Geometry: final body of the model. Coordinates: model frame, mm. Face numbers are marked on the shaded views. A direction names the side the tool comes from. Give positions to 0.01 mm unless a question says otherwise; leave off trailing zeros. Write each loop counter-clockwise with the first axis right and the second up, starting at its lowest first coordinate (ties: lowest second). Pieces come first, ordered by that corner, then holes. Notation, with made-up numbers: M -18,66 L 1,66 A17 cw 1,76 Z; hole C 9.25,-9.5 d7. An arc over 180 degrees is marked long. Use a Markdown table: item, result. Add a question column.
(1) Material intervals for L1, parallel to X at y = -2.5, z = 3; L2, parallel to X at y = 0, z = 2.5; L3, parallel to Z at x = 6.5, y = -3.5, sorted ascending.
(2) Pin query (flat end, axial travel): pin 1 Ø1 at (x, y) = (-14.5, -1.5) entering from -Z; pin 2 Ø8 at (x, z) = (20.5, 21.5) entering from -Y; pin 3 Ø1 at (x, z) = (-3.5, 25.5) entering from +Y; pin 4 Ø10 at (x, z) = (-38, 12) entering from +Y. Return the tip coordinate at first contact, or that it passes through.
(3) Cut plane A-A (y = 0). Output: boundary loops of the cut face in (x, z), plus the area to 3 significant figures.
(4) Cut plane C-C (z = 4). State how many separate pieces and enclosed holes the cut face has, plus the area to 3 significant figures.
(5) Cut plane B-B (x = -1.5). Output: boundary loops of the cut face in (y, z).
(6) Draft query along X for the marked faces 3, 4 and 5. Return one class per face: released by +X, released by -X, zero draft, split by the parting line, or undercut.
(7) Reachability of the marked faces 1 and 2 from +Z, -Z, +X, -X, +Y, -Y: full face, straight path, thin tool, end or side. Return the list, or none.
```python
from build123d import *

# Parameters (mm, degrees)
BOSS_EXTRUDE1_DEPTH             = 6.35
FILLET1_R                       = 6.35
CHAMFER1_SIZE                   = 2
SKETCH3_R                       = 2.54
CUT_EXTRUDE1_DEPTH              = 63.891530963
F_10_CLEARANCE_HOLE1_AT_2_COUNT = 2
F_10_CLEARANCE_HOLE1_AT_2_PITCH = 101.605909567
SKETCH6_R                       = 3.81
CUT_EXTRUDE2_DEPTH              = 63.891531054


with BuildPart() as part:
    # Sketch2 → Boss-Extrude1 (new, symmetric)
    with BuildSketch(Plane(origin=(0, 0, 0), x_dir=(1, 0, 0), z_dir=(0, 1, 0))):
        with BuildLine():
            Line((-27.740386752, -38.1), (27.740386752, -38.1))
            ThreePointArc((27.740386752, -38.1), (48.067233392, -23.381874086), (57.182708636, 0))
            Line((57.182708636, 0), (44.417291364, 0))
            ThreePointArc((44.417291364, 0), (38.295246108, -15.252216058), (25.367291364, -25.4))
            Line((25.367291364, -25.4), (-25.367291364, -25.4))
            ThreePointArc((-25.367291364, -25.4), (-38.295246108, -15.252216058), (-44.417291364, 0))
            Line((-44.417291364, 0), (-57.182708636, 0))
            ThreePointArc((-57.182708636, 0), (-48.067233392, -23.381874086), (-27.740386752, -38.1))
        make_face()
    extrude(amount=BOSS_EXTRUDE1_DEPTH, both=True)

    # Fillet1
    fillet1_edges = [part.edges().sort_by_distance(p)[0] for p in [
        (-25.367291364, 0, 25.4),
        (25.367291364, 0, 25.4),
        (27.740386752, 0, 38.1),
        (-27.740386752, 0, 38.1),
    ]]
    fillet(fillet1_edges, radius=FILLET1_R)

    # Chamfer1
    chamfer1_edges = [part.edges().sort_by_distance(p)[0] for p in [
        (-48.438733528, -6.35, 22.894218644),
        (38.749073181, 6.35, 14.631598188),
        (-38.749073181, -6.35, 14.631598188),
        (-38.749073181, 6.35, 14.631598188),
        (0, -6.35, 25.4),
        (0, 6.35, 25.4),
        (48.438733528, -6.35, 22.894218644),
        (48.438733528, 6.35, 22.894218644),
        (0, -6.35, 38.1),
        (-27.76741166, -6.35, 37.992751984),
        (27.76741166, -6.35, 37.992751984),
        (0, 6.35, 38.1),
        (-27.76741166, 6.35, 37.992751984),
        (27.76741166, 6.35, 37.992751984),
        (-25.4153506, -6.35, 25.238431021),
        (-25.4153506, 6.35, 25.238431021),
        (25.4153506, -6.35, 25.238431021),
        (25.4153506, 6.35, 25.238431021),
        (-48.438733528, 6.35, 22.894218644),
        (38.749073181, -6.35, 14.631598188),
    ]]
    chamfer(chamfer1_edges, length=CHAMFER1_SIZE)

    # Sketch3 → Cut-Extrude1 (cut, through all)
    with BuildSketch(Plane.XY.offset(12.7)):
        with Locations(Location((50.802954783, 0, 0), (0, 0, 180))):
            Circle(SKETCH3_R)
        with Locations(Location((-50.802954783, 0, 0), (0, 0, 180))):
            Circle(SKETCH3_R)
    extrude(amount=CUT_EXTRUDE1_DEPTH, mode=Mode.SUBTRACT)

    # Sketch5 → #10 Clearance Hole1 (revolve, cut)
    with BuildSketch(Plane(origin=(50.802954783, 0, 12.7), x_dir=(0, -1, 0), z_dir=(1, 0, 0))):
        Polygon((0, 0), (0, 12.7), (2.8067, 12.7), (2.8067, 1.0033), (3.81, 0), align=None)
    f_10_clearance_hole1 = revolve(axis=Axis((50.802954783, 0, 19.05), (0, 0, -1)), mode=Mode.SUBTRACT)

    # #10 Clearance Hole1 at 2: #10 Clearance Hole1 ×2
    with Locations(*[(-i * F_10_CLEARANCE_HOLE1_AT_2_PITCH, 0, 0) for i in range(1, F_10_CLEARANCE_HOLE1_AT_2_COUNT)]):
        add(f_10_clearance_hole1, mode=Mode.SUBTRACT)

    # Sketch6 → Cut-Extrude2 (cut, through all)
    with BuildSketch(Plane.XY.offset(12.7)):
        with Locations((50.802954783, 0)):
            Circle(SKETCH6_R)
        with Locations((-50.802954783, 0)):
            Circle(SKETCH6_R)
    extrude(amount=CUT_EXTRUDE2_DEPTH, mode=Mode.SUBTRACT)


solid = part.part
```
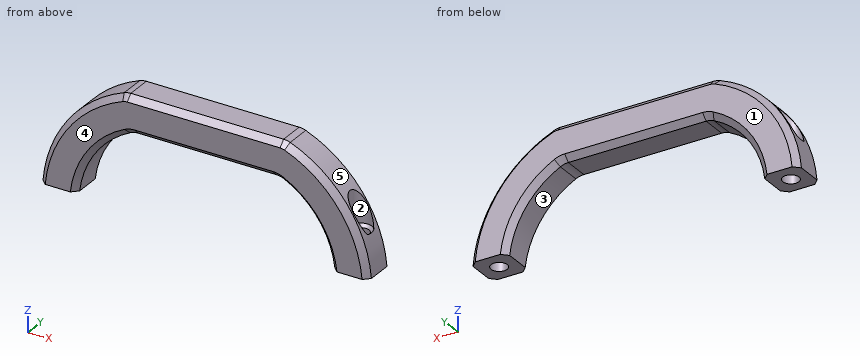
Answer list:
| question | item | result |
|---|---|---|
| 1 | L1 | -56.82 to -52.08, -49.53 to -43.91, 43.91 to 49.53, 52.08 to 56.82 |
| 1 | L2 | -56.9 to -53.61, -48 to -44.01, 44.01 to 48, 53.61 to 56.9 |
| 1 | L3 | 25.4 to 38.1 |
| 2 | pin 1 | z = 25.4 |
| 2 | pin 2 | y = -4.45 |
| 2 | pin 3 | y = 4.95 |
| 2 | pin 4 | y = 6.35 |
| 3 | outline | M -57.18,0 L -53.61,0 L -53.61,11.7 L -54.3,12.38 A44.45 ccw Z; M -48,0 L -44.42,0 A31.75 cw -26.77,24.76 A6.35 cw -23.99,25.4 L 23.99,25.4 A6.35 cw 26.77,24.76 A31.75 cw 44.42,0 L 48,0 L 48,11.7 L 46.99,12.7 L 46.99,24.72 A44.45 ccw 28.89,37.67 A6.35 ccw 26.61,38.1 L -26.61,38.1 A6.35 ccw -28.89,37.67 A44.45 ccw -46.99,24.72 L -46.99,12.7 L -48,11.7 Z; M 53.61,0 L 57.18,0 A44.45 ccw 54.3,12.38 L 53.61,11.7 Z |
| 3 | area | 1,500 mm² |
| 4 | separate pieces | 2 |
| 4 | enclosed holes | 2 |
| 4 | area | 264 mm² |
| 5 | outline | M -6.35,27.4 L -4.35,25.4 L 4.35,25.4 L 6.35,27.4 L 6.35,36.1 L 4.35,38.1 L -4.35,38.1 L -6.35,36.1 Z |
| 6 | face 3 | undercut |
| 6 | face 4 | zero draft |
| 6 | face 5 | released by +X |
| 7 | face 1 | +Z, -Z, +X, -X, +Y |
| 7 | face 2 | +Z |
